Read the model definition and answer for the solid it produces. Units are mm, in the model's axes. A direction names the side the tool comes from. Give positions to 0.01 mm unless a question says otherwise; leave off trailing zeros. Write each loop counter-clockwise with the first axis right and the second up, starting at its lowest first coordinate (ties: lowest second). Pieces come first, ordered by that corner, then holes. Notation, with made-up numbers: (-1.5, 66) -> (18.5, 66) arc R29 cw to (18.5, 91) -> close; hole circle Ø9 at (-21, 3). An arc over 180 degrees is marked (long way). Answer as CSV lines item,"result". Start each with the question number.
1. Given pin 1 (1.5 mm diameter, centred on y = 9.5, z = -75.5, fed in from +X); pin 2 (17.5 mm diameter, centred on x = -22.5, z = -52, fed in from -Y), each flat-ended and moving along its own axis, determine where each tip first touches the part or whether it passes through.
2. A tool of negligible diameter and unlimited length cuts with its end or side. For faces 4 (the flat face through (-33, 13, -3)), 5 (the flat face through (0, 15, -51)), from which of +Z, -Z, +X, -X, +Y, -Y can it reach the whole face along a straight path? Write none if from no direction.
3. The part is cut by section A-A, the plane z = -50. Determine the outline of the cut face in (x, y).
4. The part is cut by section D-D, the plane z = -86. Determine the outline of the cut face in (x, y), and give its area (3 significant figures).
5. The part is cut by section C-C, the plane y = 12. Determine the outline of the cut face in (x, z).
6. The part is cut by section B-B, the plane x = -32.5. Determine the outline of the cut face in (y, z), and give its area (3 significant figures).
7. Find the intervals of material crossed by line 1 (Z direction, x = -32.5, y = 29.15); line 2 (X direction, y = 27.75, z = -50); line 3 (Z direction, x = -26, y = 13), in increasing order.
8. For a pull along X with two mould halves and no side action, classify faces 1 (the cylindrical face through (-0.6, 15.21, -0.57)), 2 (the flat face through (-3, 13, -49)), 3 (the flat face through (-65, 15, -49)) as pulls with the +X half, pulls with the -X half, needs draft (parallel to the pull), parting line crosses it, or undercut.
Autodesk Inventor part; units mm, degrees
ref_plane "YZ Plane" through (0, 0, 0) normal (1, 0, 0) x (0, 1, 0)
ref_plane "XZ Plane" through (0, 0, 0) normal (0, 1, 0) x (-1, 0, 0)
ref_plane "XY Plane" through (0, 0, 0) normal (0, 0, 1) x (1, 0, 0)
sketch "Sketch1" plane through (0, 0, 0) normal (0, 1, 0) x (-1, 0, 0)
  line L0 (0, 0) -> (65, 0)
  line L1 (65, 0) -> (65, -100)
  line L2 (65, -100) -> (0, -100)
  line L3 (0, -100) -> (0, 0)
  line L4 (62, -3) -> (3, -3)
  line L5 (3, -3) -> (3, -97)
  line L6 (3, -97) -> (62, -97)
  line L7 (62, -97) -> (62, -3)
  dimension "d0" = 100
  dimension "d1" = 65
  dimension "d2" = 3
  dimension "d3" = 3
  dimension "d5" = 3
  dimension "d6" = 3
extrude "Extrusion1" add sketch "Sketch1" along normal blind 30
sketch "Sketch2" plane through (-62, 0, -97) normal (0, 0, 1) x (1, 0, 0)
  line L0 (62, 30) -> (-3, 30)
  line L1 (-3, 0) -> (-3, 30)
  line L2 (62, 30) -> (-3, 30)
  line L3 (-3, 30) -> (-3, 27)
  line L4 (-3, 27) -> (62, 27)
  line L5 (62, 27) -> (62, 30)
  point P0 (62, 0)
  dimension "d9" = 3
extrude "Extrusion2" add sketch "Sketch2" along normal blind 97
sketch "Sketch3" plane through (0, 30, 0) normal (0, 1, 0) x (1, 0, 0)
  circle A0 centre (-32.5, 50) radius 9
  line L0 (-65, 100) -> (-65, 0)
  line L1 (0, 0) -> (0, 100)
  line L2 (-65, 0) -> (0, 0)
  line L3 (0, 100) -> (-65, 100)
  dimension "d12" = 18
  dimension "d14" = 32.5
  dimension "d15" = 32.5
  dimension "d16" = 50
  dimension "d17" = 50
extrude "Extrusion3" cut sketch "Sketch3" against normal blind 97 contours A0
fillet "Fillet1" radius 2 4 edges at (0, 15, 0) (-65, 15, 0) (0, 15, -100) (-65, 15, -100)
equation "\"d14\" = d15"
equation "\"d16\" = d17"
properties part number "NadstavbaArduinoHranata"
Results found:
1,pin 1,"stops at x = 0"
1,pin 2,"stops at y = 27"
2,face 4,"-Y"
2,face 5,"+Z, -Z, +X, +Y, -Y"
3,outline,"(-65, 0) -> (-62, 0) -> (-62, 27) -> (-41.5, 27) -> (-41.5, 30) -> (-65, 30) -> close; (-23.5, 27) -> (-3, 27) -> (-3, 0) -> (0, 0) -> (0, 30) -> (-23.5, 30) -> close"
4,outline,"(-65, 0) -> (-62, 0) -> (-62, 27) -> (-3, 27) -> (-3, 0) -> (0, 0) -> (0, 30) -> (-65, 30) -> close"
4,area,"357 mm²"
5,outline,"(-65, -98) arc R2 ccw to (-63, -100) -> (-2, -100) arc R2 ccw to (0, -98) -> (0, -2) arc R2 ccw to (-2, 0) -> (-63, 0) arc R2 ccw to (-65, -2) -> close; hole (-62, -97) -> (-3, -97) -> (-3, -3) -> (-62, -3) -> close"
6,outline,"(0, -100) -> (30, -100) -> (30, -59) -> (27, -59) -> (27, -97) -> (0, -97) -> close; (0, -3) -> (27, -3) -> (27, -41) -> (30, -41) -> (30, 0) -> (0, 0) -> close"
6,area,"408 mm²"
7,line 1,"z = -100 to -59, -41 to 0"
7,line 2,"x = -65 to -41.5, -23.5 to 0"
7,line 3,"z = -100 to -97, -3 to 0"
8,face 1,"pulls with the +X half"
8,face 2,"undercut"
8,face 3,"pulls with the -X half"
